from build123d import *

# Parameters (mm, degrees)
BOSS_EXTRUDE1_DEPTH                         = 5
CBORE_FOR_00_BINDING_HEAD_MACHINE_S_2_COUNT = 2
CBORE_FOR_00_BINDING_HEAD_MACHINE_S_2_PITCH = 124.680760017
CBORE_FOR_00_BINDING_HEAD_MACHINE_S_3_COUNT = 2
CBORE_FOR_00_BINDING_HEAD_MACHINE_S_3_PITCH = 84.969496715
CBORE_FOR_00_BINDING_HEAD_MACHINE_S_4_COUNT = 2
CBORE_FOR_00_BINDING_HEAD_MACHINE_S_4_PITCH = 150.881103158


with BuildPart() as part:
    # Sketch2 → Boss-Extrude1 (new body)
    with BuildSketch(Plane(origin=(0, 0, 0), x_dir=(1, 0, 0), z_dir=(0, 1, 0))):
        with BuildLine():
            Line((-61, -46), (61, -46))
            ThreePointArc((61, -46), (64.535533906, -44.535533906), (66, -41))
            Line((66, -41), (66, 41))
            ThreePointArc((66, 41), (64.535533906, 44.535533906), (61, 46))
            Line((61, 46), (-61, 46))
            ThreePointArc((-61, 46), (-64.535533906, 44.535533906), (-66, 41))
            Line((-66, 41), (-66, -41))
            ThreePointArc((-66, -41), (-64.535533906, -44.535533906), (-61, -46))
        make_face()
        Polygon((-64, -33.5), (-24, -33.5), (-24, -17.5), (-15.5, -17.5), (-15.5, 19), (-24, 19), (-24, 33.5), (-64, 33.5), align=None, mode=Mode.SUBTRACT)
    extrude(amount=BOSS_EXTRUDE1_DEPTH)

    # Sketch5 → CBORE for #00 Binding Head Machine Screw1 (revolve, cut)
    with BuildSketch(Plane(origin=(-62.340407583, 5, -42.268283337), x_dir=(0, 0, 1), z_dir=(1, 0, 0))):
        Polygon((0, 0), (0, 5.396808353), (0.6604, 5), (0.6604, 0.7112), (1.5875, 0.7112), (1.5875, 0.635), (2.2225, 0), align=None)
    cbore_for_00_binding_head_machine_screw = revolve(axis=Axis((-62.340407583, 11.35, -42.268283337), (0, -1, 0)), mode=Mode.SUBTRACT)

    # CBORE for _00 Binding Head Machine S 2: CBORE for #00 Binding Head Machine Screw1 ×2
    with Locations(*[(i * CBORE_FOR_00_BINDING_HEAD_MACHINE_S_2_PITCH, 0, 0) for i in range(1, CBORE_FOR_00_BINDING_HEAD_MACHINE_S_2_COUNT)]):
        add(cbore_for_00_binding_head_machine_screw, mode=Mode.SUBTRACT)

    # CBORE for _00 Binding Head Machine S 3: CBORE for #00 Binding Head Machine Screw1 ×2
    with Locations(*[(0, 0, i * CBORE_FOR_00_BINDING_HEAD_MACHINE_S_3_PITCH) for i in range(1, CBORE_FOR_00_BINDING_HEAD_MACHINE_S_3_COUNT)]):
        add(cbore_for_00_binding_head_machine_screw, mode=Mode.SUBTRACT)

    # CBORE for _00 Binding Head Machine S 4: CBORE for #00 Binding Head Machine Screw1 ×2
    with Locations(*[Vector(0.8263510632316995, 0, 0.563155325195314) * (i * CBORE_FOR_00_BINDING_HEAD_MACHINE_S_4_PITCH) for i in range(1, CBORE_FOR_00_BINDING_HEAD_MACHINE_S_4_COUNT)]):
        add(cbore_for_00_binding_head_machine_screw, mode=Mode.SUBTRACT)


solid = part.part
Input: part model. Units: mm. Frame: model coordinates. A direction names the side the tool comes from. Coordinates: 2 decimals unless noted, no trailing zeros. Order: outer loops, then holes, each group sorted by start corner. A loop starts at its lowest first (then second) coordinate and runs counter-clockwise, first axis right, second up.
1. Contact query for flat-ended pins moving along their axis: P1, Ø1.6, axis at x = 62.5, z = 42, coming from the +Y side; P2, Ø1.6, axis at x = -63, z = -43, coming from the +Y side; P3, Ø4, axis at x = -62.34, z = -42.27, coming from the +Y side. Output: stop coordinate, or through.
Checked values:
P1: stops at y = 4.29
P2: stops at y = 4.56
P3: stops at y = 4.78
2. Draft query along X for faces 4 (the flat face through (1, 2, -46)), 5 (the flat face through (-24, 2, 26)), 6 (the flat face through (-66, 2, -1)). Return one class per face: +X half, -X half, draft (parallel to the pull), parting line (faces both ways), or undercut.
Checked values:
face 4: draft
face 5: undercut
face 6: -X half
3. Ray query, line 1 along X through (y, z) = (3.6, 20.5); line 2 along Z through (x, y) = (-41, 0.7); line 3 along X through (y, z) = (3.95, -1). Return the intervals inside material, ascending.
Checked values:
line 1: x = -66 to -64, -24 to 66
line 2: z = -46 to -33.5, 33.5 to 46
line 3: x = -66 to -64, -15.5 to 66
4. Cut plane A-A, the plane z = -12. Return loops of the section in (x, y), plus the area to 4 significant figures.
Checked values:
outline: (-66, 0) - (-64, 0) - (-64, 5) - (-66, 5) - close; (-15.5, 0) - (66, 0) - (66, 5) - (-15.5, 5) - close
area: 417.5 mm2
5. Cut plane C-C, the plane y = 1.5. Return loops of the section in (x, z), plus the area to 3 significant figures.
Checked values:
outline: (-66, -41) arc R5 ccw to (-61, -46) - (61, -46) arc R5 ccw to (66, -41) - (66, 41) arc R5 ccw to (61, 46) - (-61, 46) arc R5 ccw to (-66, 41) - close; hole (-64, -33.5) - (-24, -33.5) - (-24, -19) - (-15.5, -19) - (-15.5, 17.5) - (-24, 17.5) - (-24, 33.5) - (-64, 33.5) - close; hole circle Ø1.32 at (-62.34, -42.27); hole circle Ø1.32 at (-62.34, 42.7); hole circle Ø1.32 at (62.34, -42.27); hole circle Ø1.32 at (62.34, 42.7)
area: 9,130 mm2
6. Cut plane B-B, the plane x = -47.5. Return loops of the section in (y, z).
Checked values:
outline: (0, -46) - (5, -46) - (5, -33.5) - (0, -33.5) - close; (0, 33.5) - (5, 33.5) - (5, 46) - (0, 46) - close
7. Access query for faces 1 (the flat face through (63, 4.289, -43)), 2 (the flat face through (-20, 2, -19)), 3 (the flat face through (-1, 2, 46)). Directions: +Z, -Z, +X, -X, +Y, -Y. A direction counts if a zero-diameter tool reaches every point of the face in a straight line with its end or side. Return the directions, or none.
Checked values:
face 1: +Y
face 2: +Y, -Y
face 3: +Z, +X, -X, +Y, -Y
